from build123d import *

# Parameters (mm, degrees)
CHANFREIN1_SIZE         = 0.1
CHANFREIN1_SIZE2        = 0.111665285
CHANFREIN2_SIZE         = 0.2
CHANFREIN3_SIZE         = 0.2
TROU_TARAUD_M31_D       = 2.5
TROU_TARAUD_M31_DEPTH   = 8.5
TROU_TARAUD_M31_TIP     = 0.751075774
TROU_TARAUD_M2_51_D     = 2.05
TROU_TARAUD_M2_51_DEPTH = 8.25
TROU_TARAUD_M2_51_TIP   = 0.615882135


with BuildPart() as part:
    # Esquisse1 → Révolution1 (revolve)
    with BuildSketch(Plane.XY, mode=Mode.PRIVATE) as r_volution1_sk:
        Polygon((-14.225, 0), (-14.225, 2.025), (-4.475, 3), (3.625, 3), (3.625, 3.5), (4.625, 3.5), (4.625, 5), (7.125, 5), (7.125, 2.75), (8.425, 2.75), (8.425, 2), (14.225, 2), (14.225, 0), align=None)
    revolve(r_volution1_sk.sketch.rotate(Axis((14.225, 0, 0), (-1, 0, 0)), 90), axis=Axis((14.225, 0, 0), (-1, 0, 0)))

    # Chanfrein1
    chanfrein1_edges = [part.edges().sort_by_distance(p)[0] for p in [
        (-14.225, 0, 2.025),
    ]]
    chanfrein1_side = [part.faces().sort_by_distance(p)[0] for p in [
        (-14.225, 0, 0),
    ]]
    chamfer(chanfrein1_edges, length=CHANFREIN1_SIZE, length2=CHANFREIN1_SIZE2, reference=chanfrein1_side[0])

    # Chanfrein2
    chanfrein2_edges = [part.edges().sort_by_distance(p)[0] for p in [
        (3.625, 0, 3.5),
    ]]
    chamfer(chanfrein2_edges, length=CHANFREIN2_SIZE)

    # Chanfrein3
    chanfrein3_edges = [part.edges().sort_by_distance(p)[0] for p in [
        (7.125, 0, 5),
        (4.625, 0, 5),
        (14.225, 0, 2),
    ]]
    chamfer(chanfrein3_edges, length=CHANFREIN3_SIZE)

    # Trou taraudé M31
    with Locations(Plane.ZY.offset(14.225)):
        with Locations((0, 0)):
            Hole(TROU_TARAUD_M31_D / 2, depth=TROU_TARAUD_M31_DEPTH)
            with Locations((0, 0, -(TROU_TARAUD_M31_DEPTH + TROU_TARAUD_M31_TIP / 2))):  # 118° drill point
                Cone(0, TROU_TARAUD_M31_D / 2, TROU_TARAUD_M31_TIP, mode=Mode.SUBTRACT)

    # Trou taraudé M2.51
    with Locations(Plane(origin=(14.225, 0, 0), x_dir=(0, 0, -1), z_dir=(1, 0, 0))):
        with Locations((0, 0)):
            Hole(TROU_TARAUD_M2_51_D / 2, depth=TROU_TARAUD_M2_51_DEPTH)
            with Locations((0, 0, -(TROU_TARAUD_M2_51_DEPTH + TROU_TARAUD_M2_51_TIP / 2))):  # 118° drill point
                Cone(0, TROU_TARAUD_M2_51_D / 2, TROU_TARAUD_M2_51_TIP, mode=Mode.SUBTRACT)


solid = part.part
Geometry: final body of the model. Coordinates: model frame, mm. A direction names the side the tool comes from. Give positions to 0.01 mm unless a question says otherwise; leave off trailing zeros. Write each loop counter-clockwise with the first axis right and the second up, starting at its lowest first coordinate (ties: lowest second). Pieces come first, ordered by that corner, then holes. Notation, with made-up numbers: (3, 22) - (44, 22) arc R28 cw to (44, 47) - close; hole circle Ø5 at (4.5, 88.5). An arc over 180 degrees is marked (long way). Return JSON: item names as keys, results as strings. Group by question number.
1) Mould query, pull axis Z, two halves, no side actions, for faces 1 (the conical face through (5.466, -0.174, 0.039)), 2 (the cylindrical face through (6, 0, 5)), 3 (the flat face through (4.625, 4, 0)). Classes: released by +Z, released by -Z, zero draft, split by the parting line, or undercut.
2) First-contact query: P1, Ø6, axis at x = -1, z = -3.5, coming from the +Y side; P2, Ø1, axis at y = 2.5, z = 3.5, coming from the -X side (3 decimals); P3, Ø1.6, axis at y = 0, z = 0, coming from the -X side. Flat tips, straight axial feed; report the tip coordinate or a pass-through.
3) Line query: line 1 (Y direction, x = 8, z = 0) (3 decimals); line 2 (Y direction, x = 12.25, z = 0) (3 decimals); line 3 (X direction, y = 4.25, z = -1) (3 decimals). Output: solid intervals per line, ascending.
4) Set-up query: faces 4 (the cylindrical face through (10.042, 1.016, -0.133)), 5 (the flat face through (14.225, 1, -1)), 6 (the cylindrical face through (-9.92, -1.22, 0.27)). Return all of +Z, -Z, +X, -X, +Y, -Y with unobstructed straight access to the full face (end or side cutting, diameter ignored); none if empty.
5) Section C-C on x = -5.25. Return the cut outline in (y, z) (1 decimal).
6) Section A-A on x = -1.5. Return the cut outline in (y, z).
Filled in:
{
 "1": {"face 1": "undercut", "face 2": "split by the parting line", "face 3": "zero draft"},
 "2": {"P1": "stops at y = 2.96", "P2": "stops at x = 4.625", "P3": "stops at x = -5.45"},
 "3": {"line 1": "y = -2.75 to -1.025, 1.025 to 2.75", "line 2": "y = -2 to -1.025, 1.025 to 2", "line 3": "x = 4.625 to 7.125"},
 "4": {"face 4": "+X", "face 5": "+Z, -Z, +X, +Y, -Y", "face 6": "-X"},
 "5": {"outline": "circle Ø5.8 at (0, 0); hole circle Ø0.9 at (0, 0)"},
 "6": {"outline": "circle Ø6 at (0, 0)"}
}
